```python
from build123d import *

# Parameters (mm, degrees)
F1_DEPTH = 51.0794
F2_DEPTH = 63.5
F3_R     = 5.08


with BuildPart() as f1:
    # F0 (on Top) → F1 (new body)
    with BuildSketch(Plane.XY):
        with BuildLine():
            ThreePointArc((-14.1626298428, 3.8117302825), (-24.4520879277, 14.1355315273), (-28.2167619251, 28.2167619251))
            Line((-28.2167619251, 28.2167619251), (-55.0714641052, 28.2167619251))
            Line((-55.0714641052, 28.2167619251), (-55.0714641052, -28.2167619251))
            Line((-55.0714641052, -28.2167619251), (-28.2167619251, -28.2167619251))
            ThreePointArc((-28.2167619251, -28.2167619251), (-24.4520879277, -14.1355315273), (-14.1626298428, -3.8117302825))
            Line((-14.1626298428, -3.8117302825), (-14.1626298428, 3.8117302825))
        make_face()
        with BuildLine():
            Line((-28.2167619251, -28.2167619251), (28.2167619251, -28.2167619251))
            ThreePointArc((28.2167619251, -28.2167619251), (24.4520879277, -14.1355315273), (14.1626298428, -3.8117302825))
            Line((14.1626298428, -3.8117302825), (14.1626298428, -8.6510551789))
            ThreePointArc((14.1626298428, -8.6510551789), (18.4362835565, -10.421260508), (20.2064888856, -14.6949142218))
            ThreePointArc((20.2064888856, -14.6949142218), (14.1626298428, -20.7387732646), (8.1187707999, -14.6949142218))
            Line((8.1187707999, -14.6949142218), (-7.75476352, -14.6949142218))
            ThreePointArc((-7.75476352, -14.6949142218), (-18.6936755725, -19.2259599515), (-14.1626298428, -8.287047899))
            Line((-14.1626298428, -8.287047899), (-14.1626298428, -3.8117302825))
            ThreePointArc((-14.1626298428, -3.8117302825), (-24.4520879277, -14.1355315273), (-28.2167619251, -28.2167619251))
        make_face()
        with BuildLine():
            ThreePointArc((14.1626298428, 3.8117302825), (24.4520879277, 14.1355315273), (28.2167619251, 28.2167619251))
            Line((28.2167619251, 28.2167619251), (-28.2167619251, 28.2167619251))
            ThreePointArc((-28.2167619251, 28.2167619251), (-24.4520879277, 14.1355315273), (-14.1626298428, 3.8117302825))
            Line((-14.1626298428, 3.8117302825), (-14.1626298428, 8.0735357175))
            ThreePointArc((-14.1626298428, 8.0735357175), (-18.8446514839, 19.3769358629), (-7.5412513385, 14.6949142218))
            Line((-7.5412513385, 14.6949142218), (7.6625943184, 14.6949142218))
            ThreePointArc((7.6625943184, 14.6949142218), (14.1626298428, 21.1949497461), (20.6626653671, 14.6949142218))
            ThreePointArc((20.6626653671, 14.6949142218), (18.75884904, 10.0986950245), (14.1626298428, 8.1948786974))
            Line((14.1626298428, 8.1948786974), (14.1626298428, 3.8117302825))
        make_face()
        with BuildLine():
            Line((55.0714641052, -28.2167619251), (55.0714641052, 28.2167619251))
            Line((55.0714641052, 28.2167619251), (28.2167619251, 28.2167619251))
            ThreePointArc((28.2167619251, 28.2167619251), (24.4520879277, 14.1355315273), (14.1626298428, 3.8117302825))
            Line((14.1626298428, 3.8117302825), (14.1626298428, -3.8117302825))
            ThreePointArc((14.1626298428, -3.8117302825), (24.4520879277, -14.1355315273), (28.2167619251, -28.2167619251))
            Line((28.2167619251, -28.2167619251), (55.0714641052, -28.2167619251))
        make_face()
        with BuildLine():
            ThreePointArc((-1.8e-09, 0), (-7.3333036869, 0.9695912358), (-14.1626298428, 3.8117302825))
            Line((-14.1626298428, 3.8117302825), (-14.1626298428, -3.8117302825))
            ThreePointArc((-14.1626298428, -3.8117302825), (-7.3333036869, -0.9695912358), (-1.8e-09, 0))
        make_face()
        with BuildLine():
            Line((14.1626298428, -3.8117302825), (14.1626298428, 3.8117302825))
            ThreePointArc((14.1626298428, 3.8117302825), (7.3333036852, 0.9695912353), (-1.8e-09, 0))
            ThreePointArc((-1.8e-09, 0), (7.3333036852, -0.9695912353), (14.1626298428, -3.8117302825))
        make_face()
        with BuildLine():
            ThreePointArc((-1.8e-09, 0), (7.3333036852, 0.9695912353), (14.1626298428, 3.8117302825))
            Line((14.1626298428, 3.8117302825), (14.1626298428, 8.1948786974))
            ThreePointArc((14.1626298428, 8.1948786974), (9.5664106455, 10.0986950245), (7.6625943184, 14.6949142218))
            Line((7.6625943184, 14.6949142218), (-7.5412513385, 14.6949142218))
            ThreePointArc((-7.5412513385, 14.6949142218), (-9.4806082016, 10.0128925806), (-14.1626298428, 8.0735357175))
            Line((-14.1626298428, 8.0735357175), (-14.1626298428, 3.8117302825))
            ThreePointArc((-14.1626298428, 3.8117302825), (-7.3333036869, 0.9695912358), (-1.8e-09, 0))
        make_face()
        with BuildLine():
            ThreePointArc((14.1626298428, -3.8117302825), (7.3333036852, -0.9695912353), (-1.8e-09, 0))
            ThreePointArc((-1.8e-09, 0), (-7.3333036869, -0.9695912358), (-14.1626298428, -3.8117302825))
            Line((-14.1626298428, -3.8117302825), (-14.1626298428, -8.287047899))
            ThreePointArc((-14.1626298428, -8.287047899), (-9.631584113, -10.163868492), (-7.75476352, -14.6949142218))
            Line((-7.75476352, -14.6949142218), (8.1187707999, -14.6949142218))
            ThreePointArc((8.1187707999, -14.6949142218), (9.888976129, -10.421260508), (14.1626298428, -8.6510551789))
            Line((14.1626298428, -8.6510551789), (14.1626298428, -3.8117302825))
        make_face()
    extrude(amount=F1_DEPTH)

    # F0 (on Top) → F2 (join)
    with BuildSketch(Plane.XY):
        with BuildLine():
            Line((-28.2167619251, 28.2167619251), (28.2167619251, 28.2167619251))
            ThreePointArc((28.2167619251, 28.2167619251), (0, 56.4335238502), (-28.2167619251, 28.2167619251))
        make_face()
        with BuildLine():
            ThreePointArc((-28.2167619251, -28.2167619251), (0, -56.4335238502), (28.2167619251, -28.2167619251))
            Line((28.2167619251, -28.2167619251), (-28.2167619251, -28.2167619251))
        make_face()
    extrude(amount=F2_DEPTH)

    # F3
    f3_edges = [f1.edges().sort_by_distance(p)[0] for p in [
        (-55.071464, 0, 0),
        (-41.644113, 28.216762, 0),
        (0, 56.433524, 0),
        (41.644113, 28.216762, 0),
        (55.071464, 0, 0),
        (41.644113, -28.216762, 0),
        (0, -56.433524, 0),
        (-41.644113, -28.216762, 0),
        (0, 28.216762, 51.0794),
        (0, 28.216762, 63.5),
        (0, -28.216762, 63.5),
        (0, -28.216762, 51.0794),
        (0, -56.433524, 63.5),
        (0, 56.433524, 63.5),
        (-55.071464, -28.216762, 25.5397),
        (-55.071464, 28.216762, 25.5397),
        (-55.071464, 0, 51.0794),
        (55.071464, -28.216762, 25.5397),
        (55.071464, 0, 51.0794),
        (55.071464, 28.216762, 25.5397),
    ]]
    fillet(f3_edges, radius=F3_R)


solid = f1.part
```
For this review, take the finished solid that the model builds, in its own axes (mm). A direction names the side the tool comes from. Coordinates: 2 decimals unless noted, no trailing zeros. Order: outer loops, then holes, each group sorted by start corner. A loop starts at its lowest first (then second) coordinate and runs counter-clockwise, first axis right, second up. Notation, with made-up numbers: (34, 78.5) -> (77, 78.5) arc R21 cw to (77, 111.5) -> close; hole circle Ø1 at (16, 43). An arc over 180 degrees is marked (long way). Use CSV: the item, a comma, the result in double quotes. Start each with the question number.
Item 1: Insertion check: pin 1 (0.7 mm diameter, centred on x = -8, z = 57, fed in from +Y); pin 2 (10 mm diameter, centred on x = 22, z = 25, fed in from +Y); pin 3 (3 mm diameter, centred on y = -34.5, z = 13, fed in from -X); pin 4 (10.5 mm diameter, centred on x = -14.16, y = 14.69, fed in from +Z). Each pin has a flat end and moves straight along its axis. Give the tip position at first contact, or say it passes through.
Item 2: Wall thickness on probe 1 along Y at (x, z) = (13, 43); probe 2 along X at (y, z) = (-16, 15.5); probe 3 along Y at (x, z) = (-39, 26): over which ranges is each line inside the solid? List them lowest first.
Item 3: We need section C-C, the plane x = 0. Give the boundary of the cut face in (y, z), then the cut area to 3 significant figures.
Item 4: We need section D-D, the plane z = 49. Give the boundary of the cut face in (x, y), then the cut area to 3 significant figures.
Item 5: Draft analysis for pull direction Y (two halves, no side actions). For faces 4 (the face through (-1, 0, 51.079)), 5 (the face through (-39, -28.217, 28)), 6 (the face through (-53.62, 26.69, 28.4)), 7 (the face through (-55.071, 0, 25)), state which applies: pulls with the +Y half, pulls with the -Y half, needs draft (parallel to the pull), parting line crosses it, or undercut.
Item 6: For faces 1 (the face through (39, 28.217, 28)), 2 (the face through (-39, 28.217, 28)), 3 (the face through (-0.395, -29.665, 61.972)), list the 3-axis set-ups (+Z, -Z, +X, -X, +Y, -Y) from which the entire face can be reached by the end or side of a thin tool; tool diameter is ignored.
Item 7: We need section B-B, the plane x = 38.5. Give the boundary of the cut face in (y, z).
Item 8: We need section A-A, the plane z = 14. Give the boundary of the cut face in (x, y), then the cut area to 3 significant figures.
Derived:
1,pin 1,"stops at y = 55.38"
1,pin 2,"stops at y = 50.74"
1,pin 3,"stops at x = -27.81"
1,pin 4,"passes through"
2,probe 1,"y = -53.26 to -20.63, -8.76 to 8.3, 21.09 to 53.26"
2,probe 2,"x = -55.07 to -20.44, -7.89 to 8.26, 20.06 to 55.07"
2,probe 3,"y = -28.22 to 28.22"
3,outline,"(-56.43, 5.08) arc R5.08 ccw to (-51.35, 0) -> (51.35, 0) arc R5.08 ccw to (56.43, 5.08) -> (56.43, 58.42) arc R5.08 ccw to (51.35, 63.5) -> (33.3, 63.5) arc R5.08 ccw to (28.22, 58.42) -> (28.22, 56.16) arc R5.08 cw to (23.14, 51.08) -> (-23.14, 51.08) arc R5.08 cw to (-28.22, 56.16) -> (-28.22, 58.42) arc R5.08 ccw to (-33.3, 63.5) -> (-51.35, 63.5) arc R5.08 ccw to (-56.43, 58.42) -> close"
3,area,"6,440 mm^2"
4,outline,"(-54.09, -26.14) arc R5.08 ccw to (-49.99, -28.22) -> (-28.22, -28.22) arc R28.22 ccw to (28.22, -28.22) -> (49.99, -28.22) arc R5.08 ccw to (54.09, -26.14) -> (54.09, 26.14) arc R5.08 ccw to (49.99, 28.22) -> (28.22, 28.22) arc R28.22 ccw to (-28.22, 28.22) -> (-49.99, 28.22) arc R5.08 ccw to (-54.09, 26.14) -> close; hole circle Ø13.24 at (-14.16, 14.69); hole circle Ø12.82 at (-14.16, -14.69); hole circle Ø13 at (14.16, 14.69); hole circle Ø12.09 at (14.16, -14.69)"
4,area,"8,080 mm^2"
5,face 4,"undercut"
5,face 5,"pulls with the -Y half"
5,face 6,"pulls with the +Y half"
5,face 7,"needs draft"
6,face 1,"+Z, -Z, +X, +Y"
6,face 2,"+Z, -Z, -X, +Y"
6,face 3,"+Z, +X, -X"
7,outline,"(-28.22, 5.08) arc R5.08 ccw to (-23.14, 0) -> (23.14, 0) arc R5.08 ccw to (28.22, 5.08) -> (28.22, 51.08) -> (-28.22, 51.08) -> close"
8,outline,"(-55.07, -23.14) arc R5.08 ccw to (-49.99, -28.22) -> (-28.22, -28.22) arc R28.22 ccw to (28.22, -28.22) -> (49.99, -28.22) arc R5.08 ccw to (55.07, -23.14) -> (55.07, 23.14) arc R5.08 ccw to (49.99, 28.22) -> (28.22, 28.22) arc R28.22 ccw to (-28.22, 28.22) -> (-49.99, 28.22) arc R5.08 ccw to (-55.07, 23.14) -> close; hole circle Ø13.24 at (-14.16, 14.69); hole circle Ø12.82 at (-14.16, -14.69); hole circle Ø13 at (14.16, 14.69); hole circle Ø12.09 at (14.16, -14.69)"
8,area,"8,180 mm^2"
